```python
from build123d import *

# Parameters (mm, degrees)
SKETCH1_R           = 75
BOSS_EXTRUDE1_DEPTH = 100
BOSS_EXTRUDE2_DEPTH = 10
CHAMFER1_SIZE       = 50


with BuildPart() as part:
    # Sketch1 → Boss-Extrude1 (new body)
    with BuildSketch(Plane(origin=(0, 0, 0), x_dir=(1, 0, 0), z_dir=(0, 1, 0))):
        with Locations(Location((0, 0, 0), (0, 0, 270))):
            Circle(SKETCH1_R)
    extrude(amount=BOSS_EXTRUDE1_DEPTH)

    # Sketch2 → Boss-Extrude2 (add)
    with BuildSketch(Plane.XZ):
        with BuildLine():
            Line((-100, 12.5), (-100, -12.5))
            Line((-100, -12.5), (-73.950997289, -12.5))
            ThreePointArc((-73.950997289, -12.5), (-75, 0), (-73.950997289, 12.5))
            Line((-73.950997289, 12.5), (-100, 12.5))
        make_face()
        with BuildLine():
            ThreePointArc((75, 0), (74.737289209, -6.271969521), (73.950997289, -12.5))
            Line((73.950997289, -12.5), (100, -12.5))
            Line((100, -12.5), (100, 12.5))
            Line((100, 12.5), (73.950997289, 12.5))
            ThreePointArc((73.950997289, 12.5), (74.737289209, 6.271969521), (75, 0))
        make_face()
        with BuildLine():
            Line((-12.5, 100), (-12.5, 73.950997289))
            ThreePointArc((-12.5, 73.950997289), (0, 75), (12.5, 73.950997289))
            Line((12.5, 73.950997289), (12.5, 100))
            Line((12.5, 100), (-12.5, 100))
        make_face()
        with BuildLine():
            ThreePointArc((12.5, -73.950997289), (0, -75), (-12.5, -73.950997289))
            Line((-12.5, -73.950997289), (-12.5, -100))
            Line((-12.5, -100), (12.5, -100))
            Line((12.5, -100), (12.5, -73.950997289))
        make_face()
    extrude(amount=-BOSS_EXTRUDE2_DEPTH)

    # Chamfer1
    # the kernel refuses this chamfer: 50 mm, written as the material it adds along each edge
    with BuildSketch(Plane(origin=(0, 10, 0), x_dir=(0.9519856818942184, 0, 0.30614255089484044), z_dir=(-0.30614255089484044, 0, 0.9519856818942184))) as chamfer1_piece_1_section:
        Polygon((75, CHAMFER1_SIZE), (75 + CHAMFER1_SIZE, 0), (75, 0), align=None)
    chamfer1_piece_1 = revolve(axis=Axis((0, 10, 0), (0, 1, 0)), revolution_arc=215.653831418, mode=Mode.PRIVATE)
    chamfer1_piece_1 = split(chamfer1_piece_1, bisect_by=Plane(origin=(-12.5, 29.622120316, 1e-09), z_dir=(1, 0, 0)), keep=Keep.TOP, mode=Mode.PRIVATE)
    chamfer1_piece_1 = split(chamfer1_piece_1, bisect_by=Plane(origin=(85.193298793, 29.622120316, 12.5), z_dir=(0, 0, -1)), keep=Keep.TOP, mode=Mode.PRIVATE)
    chamfer1_piece_1 = split(chamfer1_piece_1, bisect_by=Plane(origin=(85.193298793, 29.622120316, -12.5), z_dir=(0, 0, 1)), keep=Keep.TOP, mode=Mode.PRIVATE)
    chamfer1_piece_1 = split(chamfer1_piece_1, bisect_by=Plane(origin=(100, 29.622120316, 1e-09), z_dir=(-1, 0, 0)), keep=Keep.TOP, mode=Mode.PRIVATE)
    add(chamfer1_piece_1)
    with BuildSketch(Plane(origin=(0, 10, 0), x_dir=(0.9519856818942184, 0, 0.30614255089484044), z_dir=(-0.30614255089484044, 0, 0.9519856818942184))) as chamfer1_piece_2_section:
        Polygon((75, CHAMFER1_SIZE), (75 + CHAMFER1_SIZE, 0), (75, 0), align=None)
    chamfer1_piece_2 = revolve(axis=Axis((0, 10, 0), (0, 1, 0)), revolution_arc=215.653831418, mode=Mode.PRIVATE)
    chamfer1_piece_2 = split(chamfer1_piece_2, bisect_by=Plane(origin=(12.5, 29.62212033, -85.19329881), z_dir=(-1, 0, 0)), keep=Keep.TOP, mode=Mode.PRIVATE)
    chamfer1_piece_2 = split(chamfer1_piece_2, bisect_by=Plane(origin=(-12.5, 29.62212033, -85.19329881), z_dir=(1, 0, 0)), keep=Keep.TOP, mode=Mode.PRIVATE)
    chamfer1_piece_2 = split(chamfer1_piece_2, bisect_by=Plane(origin=(0, 29.62212033, -100), z_dir=(0, 0, 1)), keep=Keep.TOP, mode=Mode.PRIVATE)
    add(chamfer1_piece_2)
    with BuildSketch(Plane(origin=(0, 10, 0), x_dir=(0.9519856818942184, 0, 0.30614255089484044), z_dir=(-0.30614255089484044, 0, 0.9519856818942184))) as chamfer1_piece_3_section:
        Polygon((75, CHAMFER1_SIZE), (75 + CHAMFER1_SIZE, 0), (75, 0), align=None)
    chamfer1_piece_3 = revolve(axis=Axis((0, 10, 0), (0, 1, 0)), revolution_arc=215.653831418, mode=Mode.PRIVATE)
    chamfer1_piece_3 = split(chamfer1_piece_3, bisect_by=Plane(origin=(-12.5, 29.622120318, 1e-09), z_dir=(-1, 0, 0)), keep=Keep.TOP, mode=Mode.PRIVATE)
    chamfer1_piece_3 = split(chamfer1_piece_3, bisect_by=Plane(origin=(-85.193298793, 29.622120318, 12.5), z_dir=(0, 0, -1)), keep=Keep.TOP, mode=Mode.PRIVATE)
    chamfer1_piece_3 = split(chamfer1_piece_3, bisect_by=Plane(origin=(-85.193298793, 29.622120318, -12.5), z_dir=(0, 0, 1)), keep=Keep.TOP, mode=Mode.PRIVATE)
    chamfer1_piece_3 = split(chamfer1_piece_3, bisect_by=Plane(origin=(-100, 29.622120318, 1e-09), z_dir=(1, 0, 0)), keep=Keep.TOP, mode=Mode.PRIVATE)
    add(chamfer1_piece_3)
    with BuildSketch(Plane(origin=(0, 10, 0), x_dir=(-0.30614255089485254, 0, 0.9519856818942145), z_dir=(-0.9519856818942145, 0, -0.30614255089485254))) as chamfer1_piece_4_section:
        Polygon((75, CHAMFER1_SIZE), (75 + CHAMFER1_SIZE, 0), (75, 0), align=None)
    chamfer1_piece_4 = revolve(axis=Axis((0, 10, 0), (0, 1, 0)), revolution_arc=215.653831418, mode=Mode.PRIVATE)
    chamfer1_piece_4 = split(chamfer1_piece_4, bisect_by=Plane(origin=(-1e-09, 29.622120316, -12.5), z_dir=(0, 0, 1)), keep=Keep.TOP, mode=Mode.PRIVATE)
    chamfer1_piece_4 = split(chamfer1_piece_4, bisect_by=Plane(origin=(12.5, 29.622120316, 85.193298793), z_dir=(-1, 0, 0)), keep=Keep.TOP, mode=Mode.PRIVATE)
    chamfer1_piece_4 = split(chamfer1_piece_4, bisect_by=Plane(origin=(-1e-09, 29.622120316, 100), z_dir=(0, 0, -1)), keep=Keep.TOP, mode=Mode.PRIVATE)
    chamfer1_piece_4 = split(chamfer1_piece_4, bisect_by=Plane(origin=(-12.5, 29.622120316, 85.193298793), z_dir=(1, 0, 0)), keep=Keep.TOP, mode=Mode.PRIVATE)
    add(chamfer1_piece_4)
    with BuildSketch(Plane(origin=(0, 10, 0), x_dir=(-0.30614255089485254, 0, 0.9519856818942145), z_dir=(-0.9519856818942145, 0, -0.30614255089485254))) as chamfer1_piece_5_section:
        Polygon((75, CHAMFER1_SIZE), (75 + CHAMFER1_SIZE, 0), (75, 0), align=None)
    chamfer1_piece_5 = revolve(axis=Axis((0, 10, 0), (0, 1, 0)), revolution_arc=215.653831418, mode=Mode.PRIVATE)
    chamfer1_piece_5 = split(chamfer1_piece_5, bisect_by=Plane(origin=(85.19329881, 29.62212033, 12.5), z_dir=(0, 0, -1)), keep=Keep.TOP, mode=Mode.PRIVATE)
    chamfer1_piece_5 = split(chamfer1_piece_5, bisect_by=Plane(origin=(85.19329881, 29.62212033, -12.5), z_dir=(0, 0, 1)), keep=Keep.TOP, mode=Mode.PRIVATE)
    chamfer1_piece_5 = split(chamfer1_piece_5, bisect_by=Plane(origin=(100, 29.62212033, 0), z_dir=(-1, 0, 0)), keep=Keep.TOP, mode=Mode.PRIVATE)
    add(chamfer1_piece_5)
    with BuildSketch(Plane(origin=(0, 10, 0), x_dir=(-0.30614255089485254, 0, 0.9519856818942145), z_dir=(-0.9519856818942145, 0, -0.30614255089485254))) as chamfer1_piece_6_section:
        Polygon((75, CHAMFER1_SIZE), (75 + CHAMFER1_SIZE, 0), (75, 0), align=None)
    chamfer1_piece_6 = revolve(axis=Axis((0, 10, 0), (0, 1, 0)), revolution_arc=215.653831418, mode=Mode.PRIVATE)
    chamfer1_piece_6 = split(chamfer1_piece_6, bisect_by=Plane(origin=(-1e-09, 29.622120318, -12.5), z_dir=(0, 0, -1)), keep=Keep.TOP, mode=Mode.PRIVATE)
    chamfer1_piece_6 = split(chamfer1_piece_6, bisect_by=Plane(origin=(12.5, 29.622120318, -85.193298793), z_dir=(-1, 0, 0)), keep=Keep.TOP, mode=Mode.PRIVATE)
    chamfer1_piece_6 = split(chamfer1_piece_6, bisect_by=Plane(origin=(-12.5, 29.622120318, -85.193298793), z_dir=(1, 0, 0)), keep=Keep.TOP, mode=Mode.PRIVATE)
    chamfer1_piece_6 = split(chamfer1_piece_6, bisect_by=Plane(origin=(-1e-09, 29.622120318, -100), z_dir=(0, 0, 1)), keep=Keep.TOP, mode=Mode.PRIVATE)
    add(chamfer1_piece_6)
    with BuildSketch(Plane(origin=(0, 10, 0), x_dir=(-0.9519928676316486, 0, -0.3061202051130742), z_dir=(0.3061202051130742, 0, -0.9519928676316486))) as chamfer1_piece_7_section:
        Polygon((75, CHAMFER1_SIZE), (75 + CHAMFER1_SIZE, 0), (75, 0), align=None)
    chamfer1_piece_7 = revolve(axis=Axis((0, 10, 0), (0, 1, 0)), revolution_arc=107.825570821, mode=Mode.PRIVATE)
    chamfer1_piece_7 = split(chamfer1_piece_7, bisect_by=Plane(origin=(-85.193298794, 29.622120316, -12.5), z_dir=(0, 0, 1)), keep=Keep.TOP, mode=Mode.PRIVATE)
    chamfer1_piece_7 = split(chamfer1_piece_7, bisect_by=Plane(origin=(-85.193298794, 29.622120316, 12.5), z_dir=(0, 0, -1)), keep=Keep.TOP, mode=Mode.PRIVATE)
    chamfer1_piece_7 = split(chamfer1_piece_7, bisect_by=Plane(origin=(-100, 29.622120316, -1e-09), z_dir=(1, 0, 0)), keep=Keep.TOP, mode=Mode.PRIVATE)
    add(chamfer1_piece_7)
    with BuildSketch(Plane(origin=(0, 10, 0), x_dir=(-0.9519928676316486, 0, -0.3061202051130742), z_dir=(0.3061202051130742, 0, -0.9519928676316486))) as chamfer1_piece_8_section:
        Polygon((75, CHAMFER1_SIZE), (75 + CHAMFER1_SIZE, 0), (75, 0), align=None)
    chamfer1_piece_8 = revolve(axis=Axis((0, 10, 0), (0, 1, 0)), revolution_arc=107.825570821, mode=Mode.PRIVATE)
    chamfer1_piece_8 = split(chamfer1_piece_8, bisect_by=Plane(origin=(-12.5, 29.622120326, 85.193298813), z_dir=(1, 0, 0)), keep=Keep.TOP, mode=Mode.PRIVATE)
    chamfer1_piece_8 = split(chamfer1_piece_8, bisect_by=Plane(origin=(-6.281740257, 29.622120326, 100), z_dir=(0, 0, -1)), keep=Keep.TOP, mode=Mode.PRIVATE)
    add(chamfer1_piece_8)
    with BuildSketch(Plane(origin=(0, 10, 0), x_dir=(0.30614255089486275, 0, -0.9519856818942113), z_dir=(0.9519856818942113, 0, 0.30614255089486275))) as chamfer1_piece_9_section:
        Polygon((75, CHAMFER1_SIZE), (75 + CHAMFER1_SIZE, 0), (75, 0), align=None)
    chamfer1_piece_9 = revolve(axis=Axis((0, 10, 0), (0, 1, 0)), revolution_arc=215.653831418, mode=Mode.PRIVATE)
    chamfer1_piece_9 = split(chamfer1_piece_9, bisect_by=Plane(origin=(1e-09, 29.622120316, 12.5), z_dir=(0, 0, -1)), keep=Keep.TOP, mode=Mode.PRIVATE)
    chamfer1_piece_9 = split(chamfer1_piece_9, bisect_by=Plane(origin=(12.5, 29.622120316, -85.193298793), z_dir=(-1, 0, 0)), keep=Keep.TOP, mode=Mode.PRIVATE)
    chamfer1_piece_9 = split(chamfer1_piece_9, bisect_by=Plane(origin=(-12.5, 29.622120316, -85.193298793), z_dir=(1, 0, 0)), keep=Keep.TOP, mode=Mode.PRIVATE)
    chamfer1_piece_9 = split(chamfer1_piece_9, bisect_by=Plane(origin=(1e-09, 29.622120316, -100), z_dir=(0, 0, 1)), keep=Keep.TOP, mode=Mode.PRIVATE)
    add(chamfer1_piece_9)
    with BuildSketch(Plane(origin=(0, 10, 0), x_dir=(0.30614255089486275, 0, -0.9519856818942113), z_dir=(0.9519856818942113, 0, 0.30614255089486275))) as chamfer1_piece_10_section:
        Polygon((75, CHAMFER1_SIZE), (75 + CHAMFER1_SIZE, 0), (75, 0), align=None)
    chamfer1_piece_10 = revolve(axis=Axis((0, 10, 0), (0, 1, 0)), revolution_arc=215.653831418, mode=Mode.PRIVATE)
    chamfer1_piece_10 = split(chamfer1_piece_10, bisect_by=Plane(origin=(-85.19329881, 29.62212033, -12.5), z_dir=(0, 0, 1)), keep=Keep.TOP, mode=Mode.PRIVATE)
    chamfer1_piece_10 = split(chamfer1_piece_10, bisect_by=Plane(origin=(-85.19329881, 29.62212033, 12.5), z_dir=(0, 0, -1)), keep=Keep.TOP, mode=Mode.PRIVATE)
    chamfer1_piece_10 = split(chamfer1_piece_10, bisect_by=Plane(origin=(-100, 29.62212033, 0), z_dir=(1, 0, 0)), keep=Keep.TOP, mode=Mode.PRIVATE)
    add(chamfer1_piece_10)
    with BuildSketch(Plane(origin=(0, 10, 0), x_dir=(0.30614255089486275, 0, -0.9519856818942113), z_dir=(0.9519856818942113, 0, 0.30614255089486275))) as chamfer1_piece_11_section:
        Polygon((75, CHAMFER1_SIZE), (75 + CHAMFER1_SIZE, 0), (75, 0), align=None)
    chamfer1_piece_11 = revolve(axis=Axis((0, 10, 0), (0, 1, 0)), revolution_arc=215.653831418, mode=Mode.PRIVATE)
    chamfer1_piece_11 = split(chamfer1_piece_11, bisect_by=Plane(origin=(1e-09, 29.622120318, 12.5), z_dir=(0, 0, 1)), keep=Keep.TOP, mode=Mode.PRIVATE)
    chamfer1_piece_11 = split(chamfer1_piece_11, bisect_by=Plane(origin=(12.5, 29.622120318, 85.193298793), z_dir=(-1, 0, 0)), keep=Keep.TOP, mode=Mode.PRIVATE)
    chamfer1_piece_11 = split(chamfer1_piece_11, bisect_by=Plane(origin=(1e-09, 29.622120318, 100), z_dir=(0, 0, -1)), keep=Keep.TOP, mode=Mode.PRIVATE)
    chamfer1_piece_11 = split(chamfer1_piece_11, bisect_by=Plane(origin=(-12.5, 29.622120318, 85.193298793), z_dir=(1, 0, 0)), keep=Keep.TOP, mode=Mode.PRIVATE)
    add(chamfer1_piece_11)
    with BuildSketch(Plane(origin=(0, 10, 0), x_dir=(0, 0, 1), z_dir=(-1, 0, 0))) as chamfer1_piece_12_section:
        Polygon((75, CHAMFER1_SIZE), (75 + CHAMFER1_SIZE, 0), (75, 0), align=None)
    chamfer1_piece_12 = revolve(axis=Axis((0, 10, 0), (0, 1, 0)), revolution_arc=107.825570821, mode=Mode.PRIVATE)
    chamfer1_piece_12 = split(chamfer1_piece_12, bisect_by=Plane(origin=(12.5, 29.622120324, 85.193298814), z_dir=(-1, 0, 0)), keep=Keep.TOP, mode=Mode.PRIVATE)
    chamfer1_piece_12 = split(chamfer1_piece_12, bisect_by=Plane(origin=(6.281740257, 29.622120324, 100), z_dir=(0, 0, -1)), keep=Keep.TOP, mode=Mode.PRIVATE)
    add(chamfer1_piece_12)
    with BuildSketch(Plane(origin=(0, 10, 0), x_dir=(0, 0, 1), z_dir=(-1, 0, 0))) as chamfer1_piece_13_section:
        Polygon((75, CHAMFER1_SIZE), (75 + CHAMFER1_SIZE, 0), (75, 0), align=None)
    chamfer1_piece_13 = revolve(axis=Axis((0, 10, 0), (0, 1, 0)), revolution_arc=107.825570821, mode=Mode.PRIVATE)
    chamfer1_piece_13 = split(chamfer1_piece_13, bisect_by=Plane(origin=(85.193298792, 29.622120318, 12.5), z_dir=(0, 0, -1)), keep=Keep.TOP, mode=Mode.PRIVATE)
    chamfer1_piece_13 = split(chamfer1_piece_13, bisect_by=Plane(origin=(85.193298792, 29.622120318, -12.5), z_dir=(0, 0, 1)), keep=Keep.TOP, mode=Mode.PRIVATE)
    chamfer1_piece_13 = split(chamfer1_piece_13, bisect_by=Plane(origin=(100, 29.622120318, -1e-09), z_dir=(-1, 0, 0)), keep=Keep.TOP, mode=Mode.PRIVATE)
    add(chamfer1_piece_13)


solid = part.part
```
Work out the finished part from the listing and answer in its coordinate system (mm). A direction names the side the tool comes from. Coordinates: 2 decimals unless noted, no trailing zeros. Loops run counter-clockwise (first coordinate to the right, second up) from the corner with the lowest first, then second, coordinate; pieces in that order, holes last. Notation, with made-up numbers: (4, 49) - (10, 49) arc R18 ccw to (10, 59) - close; hole circle Ø11 at (75.5, 38). An arc over 180 degrees is marked (long way). Use a Markdown table: item, result.
Item 1: Find section D-D, the plane y = 72. Determine the outline of the cut face in (x, z), and give its area (3 significant figures).
Evaluation:
| item | result |
|---|---|
| outline | circle Ø150 at (0, 0) |
| area | 17,700 mm2 |
Item 2: For faces 1 (the flat face through (-100, 17, 0)), 2 (the flat face through (87, 24, -12.5)), 3 (the flat face through (12.5, 23, 87)), 4 (the flat face through (-12.5, 23, 87)), 5 (the flat face through (-87, 24, -12.5)), determine the directions among +Z, -Z, +X, -X, +Y, -Y from which every point of the face is accessible in a straight line to the end or side of a thin tool.
Evaluation:
| item | result |
|---|---|
| face 1 | +Z, -Z, -X, +Y, -Y |
| face 2 | -Z, +X, +Y, -Y |
| face 3 | +Z, +X, +Y, -Y |
| face 4 | +Z, -X, +Y, -Y |
| face 5 | -Z, -X, +Y, -Y |
Item 3: Find section A-A, the plane y = 15.5. Determine the outline of the cut face in (x, z), and give its area (3 significant figures).
Evaluation:
| item | result |
|---|---|
| outline | (-100, -12.5) - (-73.95, -12.5) arc R75 ccw to (-12.5, -73.95) - (-12.5, -100) - (12.5, -100) - (12.5, -73.95) arc R75 ccw to (73.95, -12.5) - (100, -12.5) - (100, 12.5) - (73.95, 12.5) arc R75 ccw to (12.5, 73.95) - (12.5, 100) - (-12.5, 100) - (-12.5, 73.95) arc R75 ccw to (-73.95, 12.5) - (-100, 12.5) - close |
| area | 20,200 mm2 |
Item 4: Consider probe 1 along Z at (x, y) = (-82.5, 8); probe 2 along Z at (x, y) = (-21, 92.5); probe 3 along X at (y, z) = (46, -63). Determine where each line is inside the solid, lowest interval first. Write a range as from..to.
Evaluation:
| item | result |
|---|---|
| probe 1 | z = -12.5..12.5 |
| probe 2 | z = -72..72 |
| probe 3 | x = -40.69..40.69 |
Item 5: Given pin 1 Ø12 at (y, z) = (51.5, 63.5) entering from -X; pin 2 Ø21 at (y, z) = (31, -87) entering from -X; pin 3 Ø8 at (y, z) = (29, -18.5) entering from +X (3 decimals), each flat-ended and moving along its own axis, determine where each tip first touches the part or whether it passes through.
Evaluation:
| item | result |
|---|---|
| pin 1 | stops at x = -48.15 |
| pin 2 | stops at x = -12.5 |
| pin 3 | stops at x = 73.585 |
Item 6: Find section B-B, the plane z = 0. Determine the outline of the cut face in (x, y), and give its area (3 significant figures).
Evaluation:
| item | result |
|---|---|
| outline | (-100, 0) - (100, 0) - (100, 35) - (75, 60) - (75, 100) - (-75, 100) - (-75, 60) - (-100, 35) - close |
| area | 17,400 mm2 |
Item 7: Find section C-C, the plane x = 0. Determine the outline of the cut face in (y, z).
Evaluation:
| item | result |
|---|---|
| outline | (0, -100) - (35, -100) - (60, -75) - (100, -75) - (100, 75) - (60, 75) - (35, 100) - (0, 100) - close |
